```python
from build123d import *

# Parameters (mm, degrees)
SKETCH1_W           = 16
SKETCH1_H           = 34
BOSS_EXTRUDE1_DEPTH = 17
SKETCH2_W           = 24
SKETCH2_H           = 26
CUT_EXTRUDE1_DEPTH  = 3
SKETCH3_R           = 5
BOSS_EXTRUDE2_DEPTH = 1.5
BOSS_EXTRUDE3_DEPTH = 1.5


with BuildPart() as part:
    # Sketch1 → Boss-Extrude1 (new, symmetric)
    with BuildSketch(Plane(origin=(0, 23, 0), x_dir=(1, 0, 0), z_dir=(0, 1, 0))):
        Rectangle(SKETCH1_W, SKETCH1_H)
    extrude(amount=BOSS_EXTRUDE1_DEPTH, both=True)

    # Sketch2 → Cut-Extrude1 (cut, symmetric)
    with BuildSketch(Plane(origin=(-5, 0, 0), x_dir=(0, 0, -1), z_dir=(1, 0, 0))):
        with Locations((0, 23)):
            Rectangle(SKETCH2_W, SKETCH2_H)
    extrude(amount=CUT_EXTRUDE1_DEPTH, both=True, mode=Mode.SUBTRACT)

    # Sketch3 → Boss-Extrude2 (add, symmetric)
    with BuildSketch(Plane.XY.offset(18.5)):
        with Locations((0, 23)):
            Circle(SKETCH3_R)
    extrude(amount=BOSS_EXTRUDE2_DEPTH, both=True)

    # Sketch4 → Boss-Extrude3 (add, symmetric)
    with BuildSketch(Plane(origin=(0, 41.5, 0), x_dir=(1, 0, 0), z_dir=(0, 1, 0))):
        Polygon((4, 5), (4, -5), (-6, 0), align=None)
    extrude(amount=BOSS_EXTRUDE3_DEPTH, both=True)


solid = part.part
```
Check sheet for the modelled part. Datum: model origin and axes. Units: mm. A direction names the side the tool comes from. Give positions to 0.01 mm unless a question says otherwise; leave off trailing zeros. Write each loop counter-clockwise with the first axis right and the second up, starting at its lowest first coordinate (ties: lowest second). Pieces come first, ordered by that corner, then holes.
Item 1: Access from +Z, -Z, +X, -X, +Y, -Y to the whole of each face (thin tool, end or side, straight path). Record for faces 4 (the face through (-1.08, 18.12, 18.52)), 5 (the face through (-1.07, 41.521, -2.465)), 6 (the face through (-5, 23, -12)), 7 (the face through (-0.93, 41.521, 2.535)).
Item 2: Cross-section at D-D (y = 14.5). Enter the section's corners in (x, z).
Item 3: Cross-section at B-B (y = 26). Enter the section's corners in (x, z).
Item 4: Cross-section at C-C (x = 0). Enter the section's corners in (y, z), and give its area (3 significant figures).
Item 5: Cross-section at A-A (x = -6.5). Enter the section's corners in (y, z), and give its area (3 significant figures).
Item 6: Scan lines: L1, parallel to Z at x = -5.25, y = 22; L2, parallel to Y at x = -2.75, z = -8; L3, parallel to Z at x = 5.75, y = 37. Record each from-to range of solid material in increasing order.
Item 7: Gauge pin test, flat ends, axial feed: pin 1 (8 mm diameter, centred on x = 6, y = 11, fed in from +Z); pin 2 (0.9 mm diameter, centred on y = 41.5, z = 0, fed in from +X). Record the tip position at first contact, or that the pin passes through.
Item 8: Draft check along Z on faces 1 (the face through (-5, 23, 12)), 2 (the face through (0, 23, 20)), 3 (the face through (4, 42, 0)). Enter one of: released by +Z, released by -Z, zero draft, split by the parting line, or undercut.
Report:
1. face 4: +Z
1. face 5: -Z, -X, +Y
1. face 6: -X
1. face 7: +Z, -X, +Y
2. outline: (-8, -17) - (8, -17) - (8, 17) - (-8, 17) - (-8, 12) - (-2, 12) - (-2, -12) - (-8, -12) - close
3. outline: (-8, -17) - (8, -17) - (8, 17) - (4, 17) - (4, 20) - (-4, 20) - (-4, 17) - (-8, 17) - (-8, 12) - (-2, 12) - (-2, -12) - (-8, -12) - close
4. outline: (6, -17) - (40, -17) - (40, -3) - (43, -3) - (43, 3) - (40, 3) - (40, 17) - (28, 17) - (28, 20) - (18, 20) - (18, 17) - (6, 17) - close
4. area: 1,200 mm2
5. outline: (6, -17) - (40, -17) - (40, 17) - (6, 17) - close; hole (10, -12) - (36, -12) - (36, 12) - (10, 12) - close
5. area: 532 mm2
6. L1: z = -17 to -12, 12 to 17
6. L2: y = 6 to 10, 36 to 40
6. L3: z = -17 to 17
7. pin 1: stops at z = 17
7. pin 2: stops at x = 4
8. face 1: undercut
8. face 2: released by +Z
8. face 3: zero draft
